Source: CAD feature listing. Evaluate the final solid. Frame: model axes, mm. A direction names the side the tool comes from. Coordinates: 2 decimals unless noted, no trailing zeros. Loops run counter-clockwise (first coordinate to the right, second up) from the corner with the lowest first, then second, coordinate; pieces in that order, holes last. Notation, with made-up numbers: (83, -7) -> (142, -7) arc R35 ccw to (142, 27) -> close; hole circle Ø10 at (53, 63). An arc over 180 degrees is marked (long way). One line per question, with ' | ' between items. Start each with the question number.
```python
from build123d import *

# Parameters (mm, degrees)
SM_BASE_FLANGE_1_DEPTH = 12
FILLET_1_R             = 10


# Sheet-metal steps are written as plain solids
with BuildPart() as part:
    # Sketch 1 → Базовая кромка1 (new body)
    with BuildSketch(Plane(origin=(0, 0, 0), x_dir=(0, 0, -1), z_dir=(1, 0, 0))):
        with BuildLine():
            Line((0, 38.2), (0, 100))
            ThreePointArc((0, 100), (-38.268343237, -92.387953251), (70.710678119, 70.710678119))
            Line((70.710678119, 70.710678119), (27.011479041, 27.011479041))
            ThreePointArc((27.011479041, 27.011479041), (-14.618507116, -35.292198142), (0, 38.2))
        make_face()
    extrude(amount=-SM_BASE_FLANGE_1_DEPTH)

    # Скругление1
    fillet_1_edges = [part.edges().sort_by_distance(p)[0] for p in [
        (-6, 70.710678119, -70.710678119),
    ]]
    fillet(fillet_1_edges, radius=FILLET_1_R)


solid = part.part
```
(1) Access query for faces 4 (the flat face through (0, -43, 1)), 5 (the flat face through (-6, 45, -45)). Directions: +Z, -Z, +X, -X, +Y, -Y. A direction counts if a zero-diameter tool reaches every point of the face in a straight line with its end or side. Return the directions, or none.
(2) Cut plane B-B, the plane x = -2.75. Return the cut outline in (y, z), and give its area (3 significant figures).
(3) Cut plane A-A, the plane y = 0. Return the cut outline in (x, z).
(4) Draft query along Z for faces 1 (the cylindrical face through (-5.916, -88.417, 46.716)), 2 (the flat face through (-12, -43, 1)), 3 (the cylindrical face through (-6.08, 66.15, -70.99)). Return one class per face: pulls with the +Z half, pulls with the -Z half, needs draft (parallel to the pull), parting line crosses it, or undercut.
(5) Cut plane D-D, the plane z = -50. Return the cut outline in (x, y).
(6) Ray query, L1, parallel to Z at x = -4.25, y = 0; L2, parallel to Y at x = -6.5, z = 21; L3, parallel to Z at x = -4, y = -9. Return the intervals inside material, ascending.
(7) Contact query for flat-ended pins moving along their axis: pin 1 Ø5 at (x, z) = (-8, -36.5) entering from +Y; pin 2 Ø5 at (x, z) = (-3.5, -44) entering from -Y; pin 3 Ø2 at (x, y) = (-8.5, -12) entering from +Z. Output: stop coordinate, or through.
(8) Cut plane C-C, the plane z = 9. Return the cut outline in (x, y), and give its area (3 significant figures).
Here are the results:
1) face 4: +Z, -Z, +X, +Y, -Y | face 5: +X, -X, +Y
2) outline: (27.01, -27.01) arc R38.2 cw (long way) to (38.2, 0) -> (100, 0) arc R100 ccw (long way) to (62.42, -78.13) arc R10 ccw to (63.25, -63.25) -> close | area: 23,500 mm2
3) outline: (-12, -100) -> (0, -100) -> (0, -38.2) -> (-12, -38.2) -> close; (-12, 38.2) -> (0, 38.2) -> (0, 100) -> (-12, 100) -> close
4) face 1: parting line crosses it | face 2: needs draft | face 3: undercut
5) outline: (-12, -86.6) -> (0, -86.6) -> (0, 50) -> (-12, 50) -> close
6) L1: z = -100 to -38.2, 38.2 to 100 | L2: y = -97.77 to -31.91, 31.91 to 97.77 | L3: z = -99.59 to -37.12, 37.12 to 99.59
7) pin 1: stops at y = 39 | pin 2: stops at y = -90.98 | pin 3: stops at z = 99.39
8) outline: (-12, -99.59) -> (0, -99.59) -> (0, -37.12) -> (-12, -37.12) -> close; (-12, 37.12) -> (0, 37.12) -> (0, 99.59) -> (-12, 99.59) -> close | area: 1,500 mm2
